The model under review builds one solid part; all positions refer to its coordinate system, in mm. A direction names the side the tool comes from. Coordinates: 2 decimals unless noted, no trailing zeros. Loops run counter-clockwise (first coordinate to the right, second up) from the corner with the lowest first, then second, coordinate; pieces in that order, holes last. Notation, with made-up numbers: M 5,-2.75 L 19,-2.75 A21 cw 19,11.25 Z; hole C 59,32.25 d1. An arc over 180 degrees is marked long. Return JSON: item names as keys, results as strings.
```python
from build123d import *

# Parameters (mm, degrees)
SKETCH_1_W          = 22.8
SKETCH_1_H          = 32.5
EXTRUDE_1_DEPTH     = 3
SKETCH_4_R          = 1.75
CUT_EXTRUDE_2_DEPTH = 10
EXTRUDE_START       = -3
SKETCH_2_W          = 3
SKETCH_2_H          = 6
EXTRUDE_2_DEPTH     = 15.5
SKETCH_3_R          = 1.75
CUT_EXTRUDE_1_DEPTH = 27.797574517


with BuildPart() as part:
    # 草图1 → 凸台-拉伸1 (new body)
    with BuildSketch(Plane(origin=(0, 0, 0), x_dir=(1, 0, 0), z_dir=(0, 1, 0))):
        Rectangle(SKETCH_1_W, SKETCH_1_H)
    extrude(amount=EXTRUDE_1_DEPTH)

    # 草图4 → 切除-拉伸2 (cut)
    with BuildSketch(Plane(origin=(0, 3, 0), x_dir=(1, 0, 0), z_dir=(0, 1, 0))):
        with Locations(Location((-8.9, 13.75, 0), (0, 0, 270))):
            Circle(SKETCH_4_R)
        with Locations(Location((8.9, 13.75, 0), (0, 0, 270))):
            Circle(SKETCH_4_R)
        with Locations(Location((-8.9, -13.75, 0), (0, 0, 270))):
            Circle(SKETCH_4_R)
        with Locations(Location((8.9, -13.75, 0), (0, 0, 270))):
            Circle(SKETCH_4_R)
    extrude(amount=-CUT_EXTRUDE_2_DEPTH, mode=Mode.SUBTRACT)

    # 草图2 → 凸台-拉伸2 (add)
    with BuildSketch(Plane(origin=(0, 3, 0), x_dir=(1, 0, 0), z_dir=(0, 1, 0)).offset(EXTRUDE_START)):
        with Locations((-3.2, -14.5)):
            Rectangle(SKETCH_2_W, SKETCH_2_H)
        with Locations((-3.2, 14.5)):
            Rectangle(SKETCH_2_W, SKETCH_2_H)
    extrude(amount=EXTRUDE_2_DEPTH)

    # 草图3 → 切除-拉伸1 (cut, through all)
    with BuildSketch(Plane(origin=(-1.7, 0, 0), x_dir=(0, 0, -1), z_dir=(1, 0, 0))):
        with Locations((-13.85, 9.25)):
            Circle(SKETCH_3_R)
        with Locations((13.85, 9.25)):
            Circle(SKETCH_3_R)
    extrude(amount=-CUT_EXTRUDE_1_DEPTH, mode=Mode.SUBTRACT)


solid = part.part
```
1. Machinability: for faces 4 (the face through (-8, 1, -16.25)), 5 (the face through (5, 1, -16.25)), 6 (the face through (-3, 9, -11.5)), 7 (the face through (5, 1, 16.25)), which of the approach directions +Z, -Z, +X, -X, +Y, -Y give a long, thin tool a straight path to every point of the face, cutting with its end or side? Answer none if there is none.
Check values:
{"face 4": "-Z, -X, +Y, -Y", "face 5": "-Z, +X, +Y, -Y", "face 6": "+X, -X, +Y", "face 7": "+Z, +X, +Y, -Y"}
2. Add section B-B on y = 9.25. Give the boundary of the cut face in (x, z).
Check values:
{"outline": "M -4.7,-17.5 L -1.7,-17.5 L -1.7,-15.6 L -4.7,-15.6 Z; M -4.7,-12.1 L -1.7,-12.1 L -1.7,-11.5 L -4.7,-11.5 Z; M -4.7,11.5 L -1.7,11.5 L -1.7,12.1 L -4.7,12.1 Z; M -4.7,15.6 L -1.7,15.6 L -1.7,17.5 L -4.7,17.5 Z"}
3. Add section D-D on z = 13.85. Give the boundary of the cut face in (x, y), plus the area to 3 significant figures.
Check values:
{"outline": "M -11.4,0 L -10.65,0 L -10.65,3 L -11.4,3 Z; M -7.15,0 L 7.15,0 L 7.15,3 L -1.7,3 L -1.7,7.5 L -4.7,7.5 L -4.7,3 L -7.15,3 Z; M -4.7,11 L -1.7,11 L -1.7,15.5 L -4.7,15.5 Z; M 10.65,0 L 11.4,0 L 11.4,3 L 10.65,3 Z", "area": "74.4 mm²"}
4. The part is to be moulded in two halves that separate along Y. For faces 1 (the face through (-3.179, 9.776, -15.519)), 2 (the face through (-4.7, 9, 16)), 3 (the face through (0, 3, 0)), say which applies: released by +Y, released by -Y, zero draft, split by the parting line, or undercut.
Check values:
{"face 1": "undercut", "face 2": "zero draft", "face 3": "released by +Y"}
5. Add section C-C on x = -8.9. Give the boundary of the cut face in (y, z), plus the area to 3 significant figures.
Check values:
{"outline": "M 0,-16.25 L 3,-16.25 L 3,-15.5 L 0,-15.5 Z; M 0,-12 L 3,-12 L 3,12 L 0,12 Z; M 0,15.5 L 3,15.5 L 3,16.25 L 0,16.25 Z", "area": "76.5 mm²"}
6. Add section A-A on y = 12.25. Give the boundary of the cut face in (x, z).
Check values:
{"outline": "M -4.7,-17.5 L -1.7,-17.5 L -1.7,-11.5 L -4.7,-11.5 Z; M -4.7,11.5 L -1.7,11.5 L -1.7,17.5 L -4.7,17.5 Z"}
7. To check wall thickness, follow line 1 (X direction, y = 2.3, z = -13.75); line 2 (Z direction, x = -3.5, y = 3.25); line 3 (Y direction, x = -2.8, z = -13.85). State the ranges of each line that lie inside material, in increasing order.
Check values:
{"line 1": "-11.4 to -10.65, -7.15 to 7.15, 10.65 to 11.4", "line 2": "-17.5 to -11.5, 11.5 to 17.5", "line 3": "0 to 7.5, 11 to 15.5"}
8. Insertion check: pin 1 Ø3 at (x, y) = (-1, 5) entering from +Z; pin 2 Ø2.5 at (x, y) = (-7, 1) entering from -Z; pin 3 Ø4 at (x, z) = (8.9, 13.75) entering from +Y; pin 4 Ø1.8 at (y, z) = (11, -14) entering from -X. Each pin has a flat end and moves straight along its axis. Give the tip position at first contact, or say it passes through.
Check values:
{"pin 1": "z = 17.5", "pin 2": "z = -16.25", "pin 3": "y = 3", "pin 4": "x = -4.7"}
